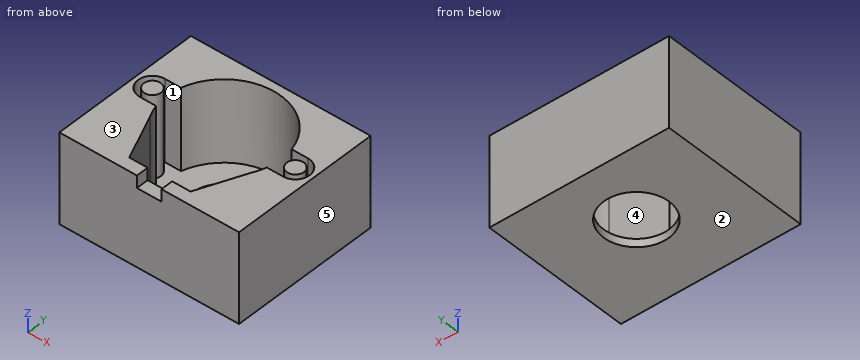
from build123d import *

# Parameters (mm, degrees)
SKETCH_1_W           = 44
SKETCH_1_H           = 37
EXTRUDE_1_DEPTH      = 22
SKETCH_2_R           = 2.1
CUT_EXTRUDE_7_DEPTH  = 20
SKETCH_13_R          = 8
CUT_EXTRUDE_11_DEPTH = 49.342527861
CUT_EXTRUDE_13_REACH = 50.343
SKETCH_15_W          = 6
SKETCH_15_H          = 3


with BuildPart() as part:
    # Sketch 1 → Extrude 1 (new body)
    with BuildSketch(Plane.XY):
        with Locations((0, 18.5)):
            Rectangle(SKETCH_1_W, SKETCH_1_H)
    extrude(amount=EXTRUDE_1_DEPTH)

    # Sketch 2 → Cut-Extrude 7 (cut)
    with BuildSketch(Plane.XY.offset(22)):
        with BuildLine():
            Line((-7.5, 3), (7.5, 3))
            Line((7.5, 3), (12.367831524, 14.439760417))
            ThreePointArc((12.367831524, 14.439760417), (13.051639376, 15.934952161), (13.555441712, 17.5))
            Line((13.555441712, 17.5), (17.5, 17.5))
            ThreePointArc((17.5, 17.5), (21, 21), (17.5, 24.5))
            Line((17.5, 24.5), (13.555441712, 24.5))
            ThreePointArc((13.555441712, 24.5), (0, 35), (-13.555441712, 24.5))
            Line((-13.555441712, 24.5), (-17.5, 24.5))
            ThreePointArc((-17.5, 24.5), (-21, 21), (-17.5, 17.5))
            Line((-17.5, 17.5), (-13.555441712, 17.5))
            ThreePointArc((-13.555441712, 17.5), (-13.051639376, 15.934952161), (-12.367831524, 14.439760417))
            Line((-12.367831524, 14.439760417), (-7.5, 3))
        make_face()
        with Locations((-17.5, 21)):
            Circle(SKETCH_2_R, mode=Mode.SUBTRACT)
        with Locations(Location((17.5, 21, 0), (0, 0, 180))):
            Circle(SKETCH_2_R, mode=Mode.SUBTRACT)
    extrude(amount=-CUT_EXTRUDE_7_DEPTH, mode=Mode.SUBTRACT)

    # Sketch 13 → Cut-Extrude 11 (cut, through all)
    with BuildSketch(Plane(origin=(0, 0, 0), x_dir=(-1, 0, 0), z_dir=(0, 0, -1))):
        with Locations((0, 20.914315439)):
            Circle(SKETCH_13_R)
    extrude(amount=-CUT_EXTRUDE_11_DEPTH, mode=Mode.SUBTRACT)

    # Sketch 15 → Cut-Extrude 13 (cut, up to next)
    with BuildSketch(Plane.XZ, mode=Mode.PRIVATE) as cut_extrude_13_sk1:
        with Locations((0, 20.5)):
            Rectangle(SKETCH_15_W, SKETCH_15_H)
    cut_extrude_13_tool1 = extrude(cut_extrude_13_sk1.sketch, amount=-CUT_EXTRUDE_13_REACH, mode=Mode.PRIVATE) & part.part
    add(cut_extrude_13_tool1.solids().sort_by_distance((0, 0, 20.5))[0], mode=Mode.SUBTRACT)


solid = part.part
Read the model definition and answer for the solid it produces. Units are mm, in the model's axes. Face numbers are marked on the shaded views. A direction names the side the tool comes from. Coordinates: 2 decimals unless noted, no trailing zeros. Write each loop counter-clockwise with the first axis right and the second up, starting at its lowest first coordinate (ties: lowest second). Pieces come first, ordered by that corner, then holes. Notation, with made-up numbers: (65.5, -19.5) -> (121.5, -19.5) arc R18 ccw to (121.5, -0.5) -> close; hole circle Ø10 at (47, 44.25). An arc over 180 degrees is marked (long way). Return JSON: item names as keys, results as strings.
(1) Each of these flat-tipped pins is pushed along its axis until it touches: P1, Ø5, axis at x = -6, y = 24.5, coming from the +Z side; P2, Ø4.5, axis at x = 16, z = 13, coming from the -Y side; P3, Ø0.9, axis at x = 0, y = 1, coming from the +Z side. Where does it stop, or does it pass through?
Answers below:
{"P1": "z = 2", "P2": "y = 0", "P3": "z = 19"}
(2) Which of the six approach directions +Z, -Z, +X, -X, +Y, -Y give full straight-line access (tool end or side, diameter ignored) to the marked faces 1 and 2?
Answers below:
{"face 1": "+Z", "face 2": "-Z, +X, -X, +Y, -Y"}
(3) The part is cut by section A-A on z = 8.25. Give the vertices of the cut face in (x, y), then the cut area to 3 significant figures.
Answers below:
{"outline": "(-22, 0) -> (22, 0) -> (22, 37) -> (-22, 37) -> close; circle Ø4.2 at (-17.5, 21); circle Ø4.2 at (17.5, 21); hole (-17.5, 17.5) -> (-13.56, 17.5) arc R14 ccw to (-12.37, 14.44) -> (-7.5, 3) -> (7.5, 3) -> (12.37, 14.44) arc R14 ccw to (13.56, 17.5) -> (17.5, 17.5) arc R3.5 ccw to (17.5, 24.5) -> (13.56, 24.5) arc R14 ccw to (-13.56, 24.5) -> (-17.5, 24.5) arc R3.5 ccw to start", "area": "854 mm^2"}
(4) The part is cut by section B-B on x = 0. Give the vertices of the cut face in (y, z), then the cut area to 3 significant figures.
Answers below:
{"outline": "(0, 0) -> (12.91, 0) -> (12.91, 2) -> (3, 2) -> (3, 19) -> (0, 19) -> close; (28.91, 0) -> (37, 0) -> (37, 22) -> (35, 22) -> (35, 2) -> (28.91, 2) -> close", "area": "133 mm^2"}
(5) For a pull along X with two mould halves and no side action, classify the marked faces 3, 4 and 5 as pulls with the +X half, pulls with the -X half, needs draft (parallel to the pull), parting line crosses it, or undercut.
Answers below:
{"face 3": "needs draft", "face 4": "undercut", "face 5": "pulls with the +X half"}
(6) The part is cut by section C-C on z = 20.75. Give the vertices of the cut face in (x, y), then the cut area to 3 significant figures.
Answers below:
{"outline": "(-22, 0) -> (-3, 0) -> (-3, 3) -> (-7.5, 3) -> (-12.37, 14.44) arc R14 cw to (-13.56, 17.5) -> (-17.5, 17.5) arc R3.5 cw to (-17.5, 24.5) -> (-13.56, 24.5) arc R14 cw to (13.56, 24.5) -> (17.5, 24.5) arc R3.5 cw to (17.5, 17.5) -> (13.56, 17.5) arc R14 cw to (12.37, 14.44) -> (7.5, 3) -> (3, 3) -> (3, 0) -> (22, 0) -> (22, 37) -> (-22, 37) -> close; circle Ø4.2 at (-17.5, 21); circle Ø4.2 at (17.5, 21)", "area": "836 mm^2"}
(7) Consider line 1 along Y through (x, z) = (0.5, 13.5); line 2 along X through (y, z) = (20.5, 14.5); line 3 along Y through (x, z) = (14, 9). Determine where each line is inside the solid, lowest interval first. Write a range as from..to.
Answers below:
{"line 1": "0..3, 34.99..37", "line 2": "-22..-20.96, -19.54..-15.46, 15.46..19.54, 20.96..22", "line 3": "0..17.5, 24.5..37"}
(8) The part is cut by section D-D on y = 2. Give the vertices of the cut face in (x, z), then the cut area to 3 significant figures.
Answers below:
{"outline": "(-22, 0) -> (22, 0) -> (22, 22) -> (3, 22) -> (3, 19) -> (-3, 19) -> (-3, 22) -> (-22, 22) -> close", "area": "950 mm^2"}
